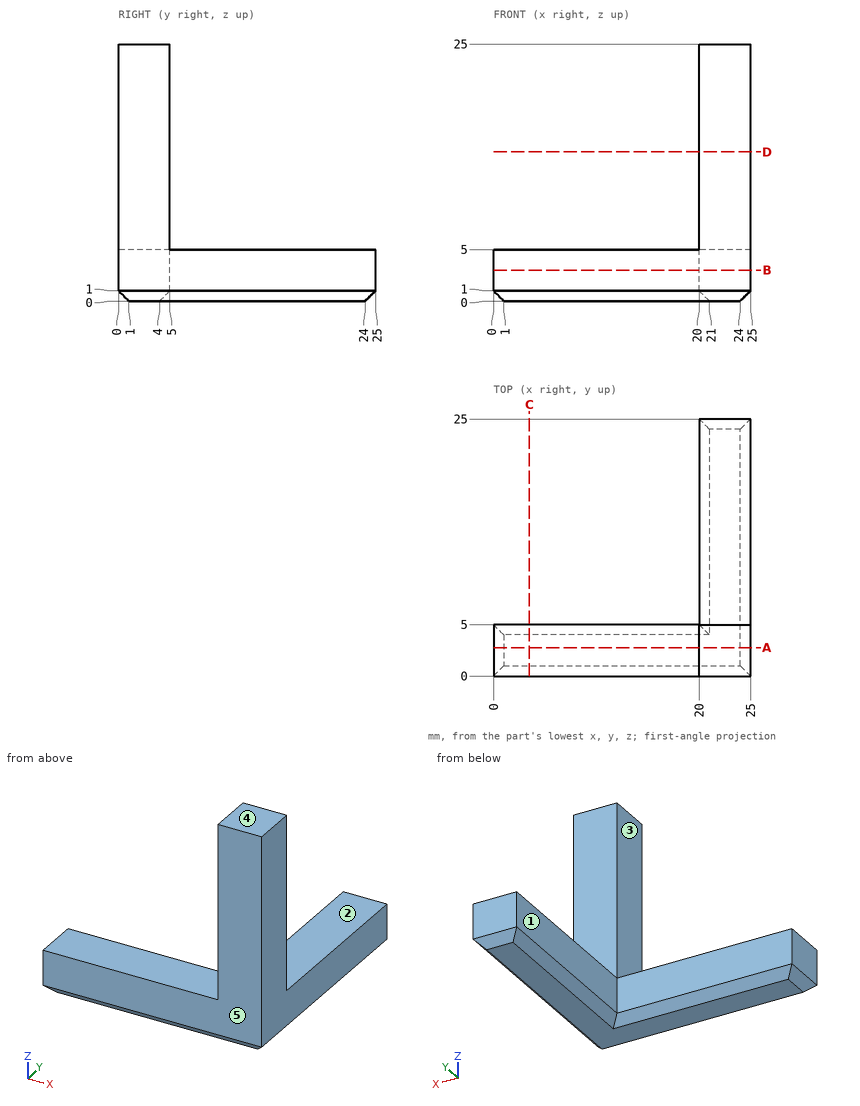
Answer from the drawing. Dimensions are ordinates in mm from the lowest x, y and z of the part. A direction names the side the tool comes from. Round coordinates to 2 decimals unless told otherwise and drop trailing zeros. Loops run counter-clockwise (first coordinate to the right, second up) from the corner with the lowest first, then second, coordinate; pieces in that order, holes last. Notation, with made-up numbers: M 55,-25 L 60,-25 A24 cw 60,-7 Z; hole C -31,82.25 d11. An arc over 180 degrees is marked long. One line per question, with ' | ' between items. Start each with the question number.
(1) A cutting plane is placed at C-C on x = 3.5. Write down the section's boundary in (y, z), plus the area to 3 significant figures.
(2) Flat-ended cylindrical pins translate along their axes: pin 1 Ø6 at (y, z) = (13, 2.5) entering from -X; pin 2 Ø4 at (x, z) = (23.5, 18) entering from +Y; pin 3 Ø12 at (x, z) = (12, 21) entering from +Y; pin 4 Ø1.5 at (x, y) = (22.5, 16.5) entering from +Z. Find the tip coordinate at first contact, or state that the pin passes through.
(3) A cutting plane is placed at B-B on z = 3. Write down the section's boundary in (x, y), plus the area to 3 significant figures.
(4) A tool of negligible diameter and unlimited length cuts with its end or side. For the marked faces 1, 2, 3, 4 and 5, from which of +Z, -Z, +X, -X, +Y, -Y can it reach the whole face along a straight path? Write none if from no direction.
(5) A cutting plane is placed at D-D on z = 14.5. Write down the section's boundary in (x, y).
(6) Find the intervals of material crossed by line 1 (X direction, y = 17.5, z = 4.75); line 2 (Y direction, x = 13, z = 4.75), in increasing order.
(7) A cutting plane is placed at A-A on y = 2.75. Write down the section's boundary in (x, z), plus the area to 3 significant figures.
Geometry check:
1) outline: M 0,1 L 1,0 L 4,0 L 5,1 L 5,5 L 0,5 Z | area: 24.0 mm²
2) pin 1: stops at x = 20 | pin 2: stops at y = 5 | pin 3: passes through | pin 4: stops at z = 5
3) outline: M 0,0 L 25,0 L 25,25 L 20,25 L 20,5 L 0,5 Z | area: 225 mm²
4) face 1: +Z, -Z, -X, +Y | face 2: +Z, +X, -X, +Y | face 3: +Z, -X, +Y, -Y | face 4: +Z, +X, -X, +Y, -Y | face 5: +Z, -Z, +X, -X, -Y
5) outline: M 20,0 L 25,0 L 25,5 L 20,5 Z
6) line 1: x = 20 to 25 | line 2: y = 0 to 5
7) outline: M 0,1 L 1,0 L 24,0 L 25,1 L 25,25 L 20,25 L 20,5 L 0,5 Z | area: 224 mm²
